For this review, take the finished solid that the model builds, in its own axes (mm). A direction names the side the tool comes from. Round coordinates to 2 decimals unless told otherwise and drop trailing zeros. Order: outer loops, then holes, each group sorted by start corner. A loop starts at its lowest first (then second) coordinate and runs counter-clockwise, first axis right, second up. Notation, with made-up numbers: (18.25, 31.5) -> (56.25, 31.5) arc R9 ccw to (56.25, 36.5) -> close; hole circle Ø2 at (-18.75, 84). An arc over 180 degrees is marked (long way). Answer in a Markdown table with one row per item.
```python
from build123d import *

# Parameters (mm, degrees)
BOSS_EXTRU_1_DEPTH = 4
ESQUISSE2_W        = 5
ESQUISSE2_H        = 2
BOSS_EXTRU_2_DEPTH = 2


with BuildPart() as part:
    # Esquisse1 → Boss.-Extru.1 (new body)
    with BuildSketch(Plane.XY):
        Polygon((21.610352861, -2.991005838), (25.610352861, -2.991005838), (25.610352861, -6.991005838), (15.610352861, -6.991005838), (15.610352861, 4.159515718), align=None)
    extrude(amount=BOSS_EXTRU_1_DEPTH)

    # Esquisse2 → Boss.-Extru.2 (add)
    with BuildSketch(Plane.XY.offset(4)):
        with Locations((18.110352861, -4.991005838)):
            Rectangle(ESQUISSE2_W, ESQUISSE2_H)
    boss_extru_2 = extrude(amount=BOSS_EXTRU_2_DEPTH)

    # Symétrie1: Boss.-Extru.2 across plane
    add(boss_extru_2.mirror(Plane.XY.offset(2)))


solid = part.part
```
Q1. Take a section at A-A, the plane x = 19.25. Write out the cut boundary in (y, z), then the cut area to 3 significant figures.
Answer key:
| item | result |
|---|---|
| outline | (-6.99, 0) -> (-5.99, 0) -> (-5.99, -2) -> (-3.99, -2) -> (-3.99, 0) -> (-0.18, 0) -> (-0.18, 4) -> (-3.99, 4) -> (-3.99, 6) -> (-5.99, 6) -> (-5.99, 4) -> (-6.99, 4) -> close |
| area | 35.3 mm^2 |
Q2. To check wall thickness, follow probe 1 along Z at (x, y) = (22.75, -6); probe 2 along Y at (x, z) = (19.25, -1.5); probe 3 along Y at (x, z) = (24.5, 0.5). State the ranges of each line that lie inside material, in increasing order.
Answer key:
| item | result |
|---|---|
| probe 1 | z = 0 to 4 |
| probe 2 | y = -5.99 to -3.99 |
| probe 3 | y = -6.99 to -2.99 |
Q3. Tool access review of faces 1 (the face through (20.61, -5, -1)), 2 (the face through (18, -5.991, -1)), 3 (the face through (20.61, -5, 5)), 4 (the face through (18, -3.991, 5)), 5 (the face through (24, -2.991, 2)): name each direction out of +Z, -Z, +X, -X, +Y, -Y from which nothing blocks a thin tool from reaching the whole face with its end or side.
Answer key:
| item | result |
|---|---|
| face 1 | -Z, +X, +Y, -Y |
| face 2 | -Z, +X, -X, -Y |
| face 3 | +Z, +X, +Y, -Y |
| face 4 | +Z, +X, -X, +Y |
| face 5 | +Z, -Z, +X, +Y |
Q4. Clearance check with flat-ended pins moving along their axes: pin 1 Ø1 at (x, z) = (17, 5) entering from +Y; pin 2 Ø1.6 at (x, z) = (17, -0.5) entering from +Y; pin 3 Ø0.6 at (y, z) = (-5.5, -1) entering from +X. State where each tip first meets the part, or that it passes through.
Answer key:
| item | result |
|---|---|
| pin 1 | stops at y = -3.99 |
| pin 2 | stops at y = 3.25 |
| pin 3 | stops at x = 20.61 |
Q5. Take a section at B-B, the plane z = 3. Write out the cut boundary in (x, y), then the cut area to 3 significant figures.
Answer key:
| item | result |
|---|---|
| outline | (15.61, -6.99) -> (25.61, -6.99) -> (25.61, -2.99) -> (21.61, -2.99) -> (15.61, 4.16) -> close |
| area | 61.5 mm^2 |
Q6. Take a section at D-D, the plane x = 21.75. Write out the cut boundary in (y, z), then the cut area to 3 significant figures.
Answer key:
| item | result |
|---|---|
| outline | (-6.99, 0) -> (-2.99, 0) -> (-2.99, 4) -> (-6.99, 4) -> close |
| area | 16.0 mm^2 |
Q7. Take a section at C-C, the plane y = -6.25. Write out the cut boundary in (x, z).
Answer key:
| item | result |
|---|---|
| outline | (15.61, 0) -> (25.61, 0) -> (25.61, 4) -> (15.61, 4) -> close |
